Verification items for the finished model (mm, model axes). Face numbers are marked on the shaded views. A direction names the side the tool comes from. Round coordinates to 2 decimals unless told otherwise and drop trailing zeros. Order: outer loops, then holes, each group sorted by start corner. A loop starts at its lowest first (then second) coordinate and runs counter-clockwise, first axis right, second up. Notation, with made-up numbers: M 87,72.5 L 130,72.5 A35 cw 130,105.5 Z; hole C 7.5,-4 d7. An arc over 180 degrees is marked long. One line per item, written item: value. Start each with the question number.
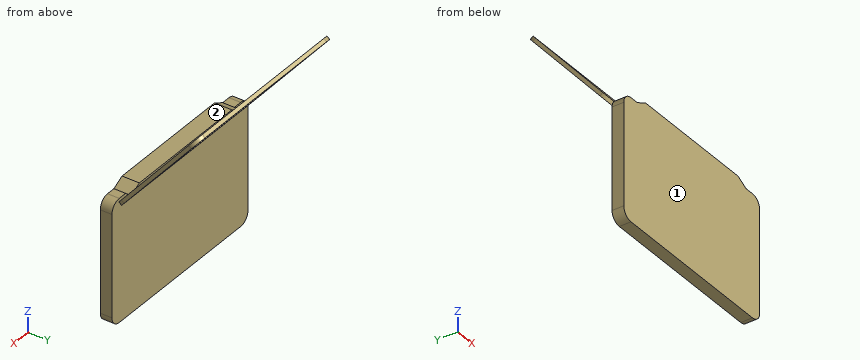
from build123d import *

# Parameters (mm, degrees)
SKETCH1_W           = 375
SKETCH1_H           = 240
BOSS_EXTRUDE1_DEPTH = 23
BOSS_EXTRUDE2_DEPTH = 34
CUT_EXTRUDE1_DEPTH  = 376
SKETCH5_W           = 375
SKETCH5_H           = 245
BOSS_EXTRUDE3_DEPTH = 7
SKETCH6_W           = 345
SKETCH6_H           = 195
CUT_EXTRUDE2_DEPTH  = 2
FILLET1_R           = 20


with BuildPart() as part:
    # Sketch1 → Boss-Extrude1 (new body)
    with BuildSketch(Plane(origin=(0, 0, 0), x_dir=(1, 0, 0), z_dir=(0, 1, 0))):
        Rectangle(SKETCH1_W, SKETCH1_H)
    extrude(amount=BOSS_EXTRUDE1_DEPTH)

    # Sketch3 → Boss-Extrude2 (add)
    with BuildSketch(Plane.XZ):
        Polygon((-150, 120), (-127.5, 132), (127.5, 132), (150, 120), align=None)
    extrude(amount=-BOSS_EXTRUDE2_DEPTH)

    # Sketch4 → Cut-Extrude1 (cut, through all)
    with BuildSketch(Plane.ZY.offset(187.5)):
        Polygon((120, 28.5), (126.554644759, 34), (120, 34), align=None)
    extrude(amount=-CUT_EXTRUDE1_DEPTH, mode=Mode.SUBTRACT)

    # Sketch5 → Boss-Extrude3 (add)
    with BuildSketch(Plane(origin=(0, -42.363978649, 35.54759886), x_dir=(-1, 0, 0), z_dir=(0, 0.766044443, -0.64278761))):
        with Locations((0, 232.74478005)):
            Rectangle(SKETCH5_W, SKETCH5_H)
    extrude(amount=BOSS_EXTRUDE3_DEPTH)

    # Sketch6 → Cut-Extrude2 (cut)
    with BuildSketch(Plane(origin=(0, -37.001667547, 31.048085592), x_dir=(1, 0, 0), z_dir=(0, 0.766044443, -0.64278761))):
        with Locations((0, -237.74478005)):
            Rectangle(SKETCH6_W, SKETCH6_H)
    extrude(amount=-CUT_EXTRUDE2_DEPTH, mode=Mode.SUBTRACT)

    # Fillet1
    fillet1_edges = [part.edges().sort_by_distance(p)[0] for p in [
        (187.5, 188.664119924, 305.43113193),
        (187.5, 31.181155551, 117.750243366),
        (-187.5, 31.181155551, 117.750243366),
        (-187.5, 188.664119924, 305.43113193),
        (-187.5, 11.5, -120),
        (187.5, 11.5, -120),
        (187.5, 11.5, 120),
        (-187.5, 11.5, 120),
    ]]
    fillet(fillet1_edges, radius=FILLET1_R)


solid = part.part
1. Depth check by flat-ended pin: pin 1 (3 mm diameter, centred on x = -34, z = 208.5, fed in from -Y); pin 2 (1.6 mm diameter, centred on x = 53, z = 129, fed in from +Y); pin 3 (9 mm diameter, centred on x = 157.5, y = 10, fed in from +Z). Enter the tip coordinate at first touch or a pass-through.
2. Section check A-A (x = -9). Record the cut outline in (y, z), and give its area (3 significant figures).
3. Scan lines: line 1 along Y through (x, z) = (156, -72); line 2 along Z through (x, y) = (-27.5, 9.5); line 3 along Z through (x, y) = (151, 19.5). Record each from-to range of solid material in increasing order.
4. Section check C-C (z = -27). Record the cut outline in (x, y), and give its area (4 significant figures).
5. Tool access check on the marked faces 1 and 2. Record the directions out of +Z, -Z, +X, -X, +Y, -Y that give a thin tool (end or side, any length) a straight path to the whole face; none if there is none.
6. Section check D-D (z = 173). Record the cut outline in (x, y), and give its area (3 significant figures).
7. Section check B-B (y = 17). Record the cut outline in (x, z).
Geometry check:
1. pin 1: stops at y = 101.5
1. pin 2: stops at y = 45.86
1. pin 3: stops at z = 120
2. outline: M 0,-120 L 23,-120 L 23,120 L 28.5,120 L 33.86,115.5 L 53.15,138.48 L 51.61,139.77 L 176.96,289.15 L 178.49,287.86 L 191.35,303.18 L 185.98,307.68 L 34,126.55 L 34,132 L 0,132 Z
2. area: 7,230 mm²
3. line 1: y = 0 to 23
3. line 2: z = -120 to 132
3. line 3: z = -120 to 120
4. outline: M -187.5,0 L 187.5,0 L 187.5,23 L -187.5,23 Z
4. area: 8,625 mm²
5. face 1: +Z, -Z, +X, -X, -Y
5. face 2: +Z, +X, -X, -Y
6. outline: M -187.5,72.97 L 187.5,72.97 L 187.5,82.11 L 172.5,82.11 L 172.5,79.5 L -172.5,79.5 L -172.5,82.11 L -187.5,82.11 Z
6. area: 2,530 mm²
7. outline: M -187.5,-100 A20 ccw -167.5,-120 L 167.5,-120 A20 ccw 187.5,-100 L 187.5,100 A20 ccw 167.5,120 L 150,120 L 127.5,132 L -127.5,132 L -150,120 L -167.5,120 A20 ccw -187.5,100 Z
